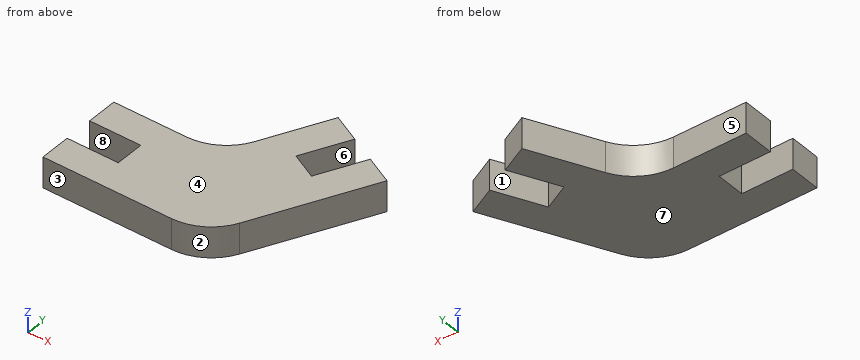
```python
from build123d import *

# Parameters (mm, degrees)
F1_DEPTH = 3


with BuildPart() as f1:
    # F0 (on Top) → F1 (new body)
    with BuildSketch(Plane.XY):
        with BuildLine():
            Line((-7.495554, -1.252463), (-2.495554, -1.252463))
            Line((-2.495554, -1.252463), (-2.495554, -4.052463))
            Line((-2.495554, -4.052463), (-7.495554, -4.052463))
            Line((-7.495554, -4.052463), (-7.495554, -7.052463))
            Line((-7.495554, -7.052463), (5.053015, -7.052463))
            ThreePointArc((5.053015, -7.052463), (7.682229, -6.305372), (9.525738, -4.287356))
            Line((9.525738, -4.287356), (15.134679, 6.937898))
            Line((15.134679, 6.937898), (12.451045, 8.278834))
            Line((12.451045, 8.278834), (10.216152, 3.806111))
            Line((10.216152, 3.806111), (7.711427, 5.057651))
            Line((7.711427, 5.057651), (9.94632, 9.530374))
            Line((9.94632, 9.530374), (7.262687, 10.87131))
            Line((7.262687, 10.87131), (4.085441, 4.512644))
            ThreePointArc((4.085441, 4.512644), (2.241932, 2.494628), (-0.387282, 1.747537))
            Line((-0.387282, 1.747537), (-7.495554, 1.747537))
            Line((-7.495554, 1.747537), (-7.495554, -1.252463))
        make_face()
    extrude(amount=F1_DEPTH)


solid = f1.part
```
Source: CAD feature listing. Evaluate the final solid. Frame: model axes, mm. Face numbers are marked on the shaded views. A direction names the side the tool comes from. Round coordinates to 2 decimals unless told otherwise and drop trailing zeros. Loops run counter-clockwise (first coordinate to the right, second up) from the corner with the lowest first, then second, coordinate; pieces in that order, holes last. Notation, with made-up numbers: M 6,-13 L 11,-13 A33 cw 11,25 Z; hole C 85,-26.75 d5. An arc over 180 degrees is marked long. Use a Markdown table: item, result. Add a question column.
1. Contact query for flat-ended pins moving along their axis: P1, Ø2, axis at x = -4, y = 4.5, coming from the +Z side; P2, Ø1.5, axis at x = -4, z = 1.5, coming from the +Y side; P3, Ø1, axis at x = 10, z = 2, coming from the +Y side; P4, Ø1.4, axis at y = -2.5, z = 1, coming from the -X side. Output: stop coordinate, or through.
2. Mould query, pull axis X, two halves, no side actions, for the marked faces 1, 2 and 3. Classes: pulls with the +X half, pulls with the -X half, needs draft (parallel to the pull), parting line crosses it, or undercut.
3. Reachability of the marked faces 4, 5, 6, 7 and 8 from +Z, -Z, +X, -X, +Y, -Y: full face, straight path, thin tool, end or side. Return the list, or none.
4. Section query B-B on z = 1.75. Return the cut outline in (x, y).
5. Section query D-D on y = 1.5. Return the cut outline in (x, z), then the cut area to 3 significant figures.
6. Section query A-A on x = -3.25. Return the cut outline in (y, z).
7. Section query C-C on y = 7.5. Return the cut outline in (x, z), then the cut area to 3 significant figures.
8. Line query: line 1 (Y direction, x = -2.25, z = 0.7); line 2 (X direction, y = 6.25, z = 2.3); line 3 (Y direction, x = 8.25, z = 1.5). Output: solid intervals per line, ascending.
Reported:
| question | item | result |
|---|---|---|
| 1 | P1 | passes through |
| 1 | P2 | stops at y = 1.75 |
| 1 | P3 | stops at y = 9.75 |
| 1 | P4 | stops at x = -2.5 |
| 2 | face 1 | undercut |
| 2 | face 2 | pulls with the +X half |
| 2 | face 3 | needs draft |
| 3 | face 4 | +Z, +X, -X, +Y, -Y |
| 3 | face 5 | +Z, -Z, -X, +Y |
| 3 | face 6 | +Z, -Z |
| 3 | face 7 | -Z, +X, -X, +Y, -Y |
| 3 | face 8 | +Z, -Z, -X |
| 4 | outline | M -7.5,-7.05 L 5.05,-7.05 A5 ccw 9.53,-4.29 L 15.13,6.94 L 12.45,8.28 L 10.22,3.81 L 7.71,5.06 L 9.95,9.53 L 7.26,10.87 L 4.09,4.51 A5 cw -0.39,1.75 L -7.5,1.75 L -7.5,-1.25 L -2.5,-1.25 L -2.5,-4.05 L -7.5,-4.05 Z |
| 5 | outline | M -7.5,0 L 12.42,0 L 12.42,3 L -7.5,3 Z |
| 5 | area | 59.7 mm² |
| 6 | outline | M -7.05,0 L -4.05,0 L -4.05,3 L -7.05,3 Z; M -1.25,0 L 1.75,0 L 1.75,3 L -1.25,3 Z |
| 7 | outline | M 5.58,0 L 8.93,0 L 8.93,3 L 5.58,3 Z; M 12.06,0 L 14.01,0 L 14.01,3 L 12.06,3 Z |
| 7 | area | 15.9 mm² |
| 8 | line 1 | y = -7.05 to 1.75 |
| 8 | line 2 | x = 4.95 to 8.31, 11.44 to 14.79 |
| 8 | line 3 | y = -5.9 to 4.79, 6.14 to 10.38 |
